```python
from build123d import *

# Parameters (mm, degrees)
F0_R      = 45.212
F1_DEPTH  = 12.065
F2_R      = 2.5908
F3_DEPTH  = 25.4
F4_R      = 14.5415
F5_DEPTH  = 25.4
F7_DEPTH  = 9.525
F8_R      = 15.24
F9_DEPTH  = 12.065
F10_R     = 14.351
F11_DEPTH = 35.56
F12_R     = 5.08
F13_DEPTH = 38.1


# Not quite as in the source:
# - a feature names something its author has since deleted; it is built from what else it names


with BuildPart() as f1:
    # F0 (on Top) → F1 (new body)
    with BuildSketch(Plane.XY):
        Circle(F0_R)
    extrude(amount=F1_DEPTH)

    # F2 (on face) → F3 (cut)
    with BuildSketch(Plane.XY.offset(12.065)):
        with Locations((-6.1631285115, 23.0011087385)):
            Circle(F2_R)
        with Locations((-23.0011087385, 6.1631285115)):
            Circle(F2_R)
        with Locations((-16.837980227, -16.837980227)):
            Circle(F2_R)
        with Locations((6.1631285115, -23.0011087385)):
            Circle(F2_R)
        with Locations((23.0011087385, -6.1631285115)):
            Circle(F2_R)
        with Locations((16.837980227, 16.837980227)):
            Circle(F2_R)
    extrude(amount=-F3_DEPTH, mode=Mode.SUBTRACT)

    # F4 (on face) → F5 (cut)
    with BuildSketch(Plane.XY.offset(12.065)):
        Circle(F4_R)
    extrude(amount=-F5_DEPTH, mode=Mode.SUBTRACT)

    # F6 (on face) → F7 (cut)
    with BuildSketch(Plane.XY.offset(12.065)):
        Polygon((-4.7398149494, 28.3129872672), (-10.0516934782, 26.8896737052), (-11.4750070402, 21.5777951764), (-7.5864420736, 17.6892302098), (-2.2745635448, 19.1125437718), (-0.8512499828, 24.4244223006), align=None)
        Polygon((22.1498587557, 18.2612937891), (18.2612937891, 22.1498587557), (12.9494152603, 20.7265451937), (11.5261016983, 15.4146666649), (15.4146666649, 11.5261016983), (20.7265451937, 12.9494152603), align=None)
        Polygon((26.8896737052, -10.0516934782), (28.3129872672, -4.7398149494), (24.4244223006, -0.8512499828), (19.1125437718, -2.2745635448), (17.6892302098, -7.5864420736), (21.5777951764, -11.4750070402), align=None)
        Polygon((4.7398149494, -28.3129872672), (10.0516934782, -26.8896737052), (11.4750070402, -21.5777951764), (7.5864420736, -17.6892302098), (2.2745635448, -19.1125437718), (0.8512499828, -24.4244223006), align=None)
        Polygon((-22.1498587557, -18.2612937891), (-18.2612937891, -22.1498587557), (-12.9494152603, -20.7265451937), (-11.5261016983, -15.4146666649), (-15.4146666649, -11.5261016983), (-20.7265451937, -12.9494152603), align=None)
        Polygon((-26.8896737052, 10.0516934782), (-28.3129872672, 4.7398149494), (-24.4244223006, 0.8512499828), (-19.1125437718, 2.2745635448), (-17.6892302098, 7.5864420736), (-21.5777951764, 11.4750070402), align=None)
    extrude(amount=-F7_DEPTH, mode=Mode.SUBTRACT)

    # F8 (on face) → F9 (join)
    with BuildSketch(Plane.XY.offset(12.065)):
        Circle(F8_R)
    extrude(amount=-F9_DEPTH)

    # F10 (on face) → F11 (join)
    with BuildSketch(Plane.XY.offset(12.065)):
        Circle(F10_R)
    extrude(amount=-F11_DEPTH)

    # F12 (on face) → F13 (cut)
    with BuildSketch(Plane.XY.offset(12.065)):
        Circle(F12_R)
    extrude(amount=-F13_DEPTH, mode=Mode.SUBTRACT)


solid = f1.part
```
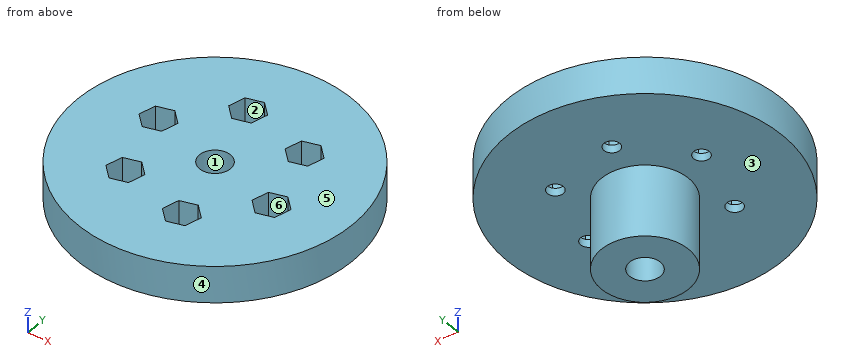
The model under review builds one solid part; all positions refer to its coordinate system, in mm. Face numbers are marked on the shaded views. A direction names the side the tool comes from. Round coordinates to 2 decimals unless told otherwise and drop trailing zeros. Loops run counter-clockwise (first coordinate to the right, second up) from the corner with the lowest first, then second, coordinate; pieces in that order, holes last. Notation, with made-up numbers: M 79,23.25 L 88,23.25 A21 ccw 88,50.25 Z; hole C -37,-12 d10. An arc over 180 degrees is marked long. Answer as a JSON object with one key per item and string values.
(1) Draft analysis for pull direction X (two halves, no side actions). For the marked faces 4, 5 and 6, state which applies: released by +X, released by -X, zero draft, split by the parting line, or undercut.
Resolved:
{"face 4": "split by the parting line", "face 5": "zero draft", "face 6": "undercut"}
(2) Take a section at C-C on x = 39. Give the boundary of the cut face in (y, z) (3 decimals).
Resolved:
{"outline": "M -22.872,0 L 22.872,0 L 22.872,12.065 L -22.872,12.065 Z"}
(3) Tool access review of the marked faces 1, 2 and 3: name each direction out of +Z, -Z, +X, -X, +Y, -Y from which nothing blocks a thin tool from reaching the whole face with its end or side.
Resolved:
{"face 1": "+Z, -Z", "face 2": "+Z", "face 3": "-Z"}
(4) Take a section at A-A on z = -17.5. Give the boundary of the cut face in (x, y).
Resolved:
{"outline": "C 0,0 d28.7; hole C 0,0 d10.16"}
(5) Clearance check with flat-ended pins moving along their axes: P1, Ø8.5, axis at x = 16.84, y = 16.84, coming from the +Z side; P2, Ø8.5, axis at x = -23, y = 6.16, coming from the -Z side; P3, Ø8, axis at x = -16, z = -16.5, coming from the +Y side; P4, Ø4, axis at x = 23, y = -6.16, coming from the +Z side. State where each tip first meets the part, or that it passes through.
Resolved:
{"P1": "z = 2.54", "P2": "z = 0", "P3": "y = 7.87", "P4": "through"}
(6) To check wall thickness, follow line 1 along Z through (x, y) = (23.5, -32.5) (3 decimals); line 2 along Y through (x, z) = (8, 8); line 3 along Y through (x, z) = (26, 3.5). State the ranges of each line that lie inside material, in increasing order.
Resolved:
{"line 1": "0 to 12.065", "line 2": "-44.5 to -27.44, -18.1 to 44.5", "line 3": "-36.99 to -10.29, -2.43 to 36.99"}
(7) Take a section at B-B on z = 4. Count the separate pieces of the cut face and the enclosed holes in it, and give its area (3 significant figures).
Resolved:
{"separate pieces": "1", "enclosed holes": "7", "area": "5,870 mm²"}
(8) Take a section at D-D on y = -34. Give the boundary of the cut face in (x, z) (3 decimals), and give its area (3 significant figures).
Resolved:
{"outline": "M -29.801,0 L 29.801,0 L 29.801,12.065 L -29.801,12.065 Z", "area": "719 mm²"}
